For this review, use the dimensioned drawing (mm, ordinates from the lowest corner) and the shaded views. A direction names the side the tool comes from. Round coordinates to 2 decimals unless told otherwise and drop trailing zeros. Loops run counter-clockwise (first coordinate to the right, second up) from the corner with the lowest first, then second, coordinate; pieces in that order, holes last. Notation, with made-up numbers: (49.5, 4) - (92.5, 4) arc R17 ccw to (92.5, 29) - close; hole circle Ø3 at (79.25, 82). An arc over 180 degrees is marked (long way). Answer as CSV lines item,"result". Start each with the question number.
(1) Consider section B-B (z = 16.11). Give the boundary of the cut face in (x, y), and give its area (3 significant figures).
(2) Consider section A-A (x = 3). Give the boundary of the cut face in (y, z).
(3) Wall thickness on L1, parallel to X at y = 0.7, z = 16.11; L2, parallel to X at y = 27.5, z = 50; L3, parallel to X at y = 20.5, z = 43.5: over which ranges is each line inside the solid? List them lowest first.
(4) Consider section C-C (z = 41.59). Give the boundary of the cut face in (x, y).
(5) Mouldability with a two-part tool opening along Z and no side actions: class the marked faces 4 and 5 as released by +Z, released by -Z, zero draft, split by the parting line, or undercut.
(6) Consider section D-D (y = 22.93). Give the boundary of the cut face in (x, z).
(7) For P1, Ø12, axis at y = 7, z = 8, coming from the +X side; P2, Ø6, axis at y = 8, z = 38, coming from the -X side; P3, Ø10.5, axis at x = 15, z = 18.5, coming from the +Y side; P4, Ø3, axis at x = 3, z = 16.11, coming from the +Y side, all flat-tipped, find the tip position at first contact; note any pin that passes through.
(8) For the marked faces 1, 2 and 3, list the 3-axis set-ups (+Z, -Z, +X, -X, +Y, -Y) from which the entire face can be reached by the end or side of a thin tool; tool diameter is ignored.
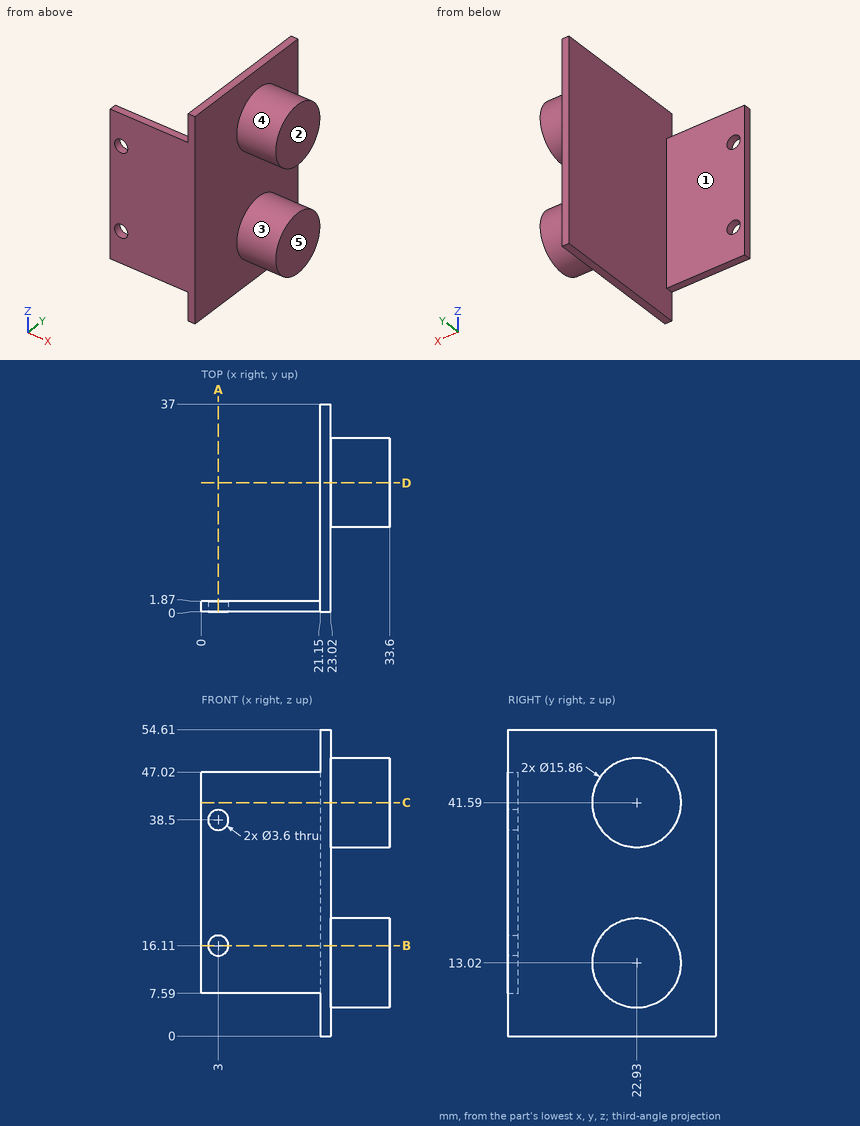
Determined:
1,outline,"(0, 0) - (1.2, 0) - (1.2, 1.87) - (0, 1.87) - close; (4.8, 0) - (23.02, 0) - (23.02, 15.63) - (33.6, 15.63) - (33.6, 30.23) - (23.02, 30.23) - (23.02, 37) - (21.15, 37) - (21.15, 1.87) - (4.8, 1.87) - close"
1,area,"257 mm^2"
2,outline,"(0, 7.59) - (1.87, 7.59) - (1.87, 14.31) - (0, 14.31) - close; (0, 17.91) - (1.87, 17.91) - (1.87, 36.7) - (0, 36.7) - close; (0, 40.3) - (1.87, 40.3) - (1.87, 47.02) - (0, 47.02) - close"
3,L1,"x = 0 to 1.2, 4.8 to 23.02"
3,L2,"x = 21.15 to 23.02"
3,L3,"x = 21.15 to 33.6"
4,outline,"(0, 0) - (23.02, 0) - (23.02, 15) - (33.6, 15) - (33.6, 30.86) - (23.02, 30.86) - (23.02, 37) - (21.15, 37) - (21.15, 1.87) - (0, 1.87) - close"
5,face 4,"undercut"
5,face 5,"zero draft"
6,outline,"(21.15, 0) - (23.02, 0) - (23.02, 5.09) - (33.6, 5.09) - (33.6, 20.95) - (23.02, 20.95) - (23.02, 33.66) - (33.6, 33.66) - (33.6, 49.52) - (23.02, 49.52) - (23.02, 54.61) - (21.15, 54.61) - close"
7,P1,"stops at x = 23.02"
7,P2,"stops at x = 21.15"
7,P3,"stops at y = 1.87"
7,P4,"passes through"
8,face 1,"+Z, -Z, -X, +Y"
8,face 2,"+Z, -Z, +X, +Y, -Y"
8,face 3,"+X"
